```python
from build123d import *

# Parameters (mm, degrees)
SKETCH009_W     = 12.5
SKETCH009_H     = 5.72
PAD007_DEPTH    = 6.75
PAD008_DEPTH    = 0.5
POCKET002_DEPTH = 12


with BuildPart() as part:
    # Sketch009 → Pad007 (new body, symmetric)
    with BuildSketch(Plane.XZ):
        with Locations((0, 4.14)):
            Rectangle(SKETCH009_W, SKETCH009_H)
    extrude(amount=PAD007_DEPTH, both=True)

    # Sketch010 (on Face6 of Pad007) → Pad008 (join)
    with BuildSketch(Plane.XZ.offset(6.75)):
        with BuildLine():
            ThreePointArc((-6.75, 7.74), (-7.103553, 7.593553), (-7.25, 7.24))
            Line((-7.25, 1.04), (-7.25, 7.24))
            ThreePointArc((-7.25, 1.04), (-7.103553, 0.686447), (-6.75, 0.54))
            Line((6.75, 0.54), (-6.75, 0.54))
            ThreePointArc((6.75, 0.54), (7.103553, 0.686447), (7.25, 1.04))
            Line((7.25, 7.24), (7.25, 1.04))
            ThreePointArc((7.25, 7.24), (7.103553, 7.593553), (6.75, 7.74))
            Line((-6.75, 7.74), (6.75, 7.74))
        make_face()
    extrude(amount=PAD008_DEPTH)

    # Sketch011 (on Face5 of Pad008) → Pocket002 (cut)
    with BuildSketch(Plane.XZ.offset(7.25)):
        with BuildLine():
            ThreePointArc((-5.35, 6.29), (-5.703553, 6.143553), (-5.85, 5.79))
            Line((-5.85, 2.49), (-5.85, 5.79))
            ThreePointArc((-5.85, 2.49), (-5.703553, 2.136447), (-5.35, 1.99))
            Line((5.35, 1.99), (-5.35, 1.99))
            ThreePointArc((5.35, 1.99), (5.703553, 2.136447), (5.85, 2.49))
            Line((5.85, 5.79), (5.85, 2.49))
            ThreePointArc((5.85, 5.79), (5.703553, 6.143553), (5.35, 6.29))
            Line((-5.35, 6.29), (5.35, 6.29))
        make_face()
    extrude(amount=-POCKET002_DEPTH, mode=Mode.SUBTRACT)


with BuildPart() as part_1:
    # Body004 placement: moved
    add(part.part.moved(Location((-9.53, -23.5, 1.6))))


solid = part_1.part
```
Work out the finished part from the listing and answer in its coordinate system (mm). A direction names the side the tool comes from. Coordinates: 2 decimals unless noted, no trailing zeros. Write each loop counter-clockwise with the first axis right and the second up, starting at its lowest first coordinate (ties: lowest second). Pieces come first, ordered by that corner, then holes. Notation, with made-up numbers: (-38.75, 62.5) - (13.25, 62.5) arc R18 ccw to (13.25, 92.5) - close; hole circle Ø6 at (55, 38.25). An arc over 180 degrees is marked (long way). Answer as a JSON object with one key per item and string values.
Q1. Consider L1, parallel to Z at x = -14.25, y = -25.5; L2, parallel to X at y = -29.75, z = 5.5; L3, parallel to X at y = -26.25, z = 3.25. Determine where each line is inside the solid, lowest interval first. Write a range as from..to.
Results list:
{"L1": "z = 2.88..3.59, 7.89..8.6", "L2": "x = -15.78..-15.38, -3.68..-3.28", "L3": "x = -15.78..-3.28"}
Q2. Find section B-B (z = 4.5). Write down the section's boundary in (x, y), plus the area to 3 significant figures.
Results list:
{"outline": "(-16.78, -30.75) - (-15.38, -30.75) - (-15.38, -18.75) - (-3.68, -18.75) - (-3.68, -30.75) - (-2.28, -30.75) - (-2.28, -30.25) - (-3.28, -30.25) - (-3.28, -16.75) - (-15.78, -16.75) - (-15.78, -30.25) - (-16.78, -30.25) - close", "area": "35.6 mm^2"}
Q3. Find section D-D (y = -18). Write down the section's boundary in (x, z), plus the area to 3 significant figures.
Results list:
{"outline": "(-15.78, 2.88) - (-3.28, 2.88) - (-3.28, 8.6) - (-15.78, 8.6) - close", "area": "71.5 mm^2"}
Q4. Which of the six approach directions +Z, -Z, +X, -X, +Y, -Y give full straight-line access (tool end or side, diameter ignored) to faces 1 (the flat face through (-15.78, -24, 6)), 2 (the flat face through (-10, -25, 7.89)), 3 (the flat face through (-3.28, -24, 6)), 4 (the flat face through (-10, -24, 2.88))?
Results list:
{"face 1": "+Z, -Z, -X, +Y", "face 2": "-Y", "face 3": "+Z, -Z, +X, +Y", "face 4": "-Z, +X, -X, +Y"}
Q5. For a pull along Z with two mould halves and no side action, classify faces 5 (the flat face through (-10, -24, 8.6)), 6 (the flat face through (-10, -30.25, 9)), 7 (the flat face through (-15.38, -25, 6)) as pulls with the +Z half, pulls with the -Z half, needs draft (parallel to the pull), parting line crosses it, or undercut.
Results list:
{"face 5": "pulls with the +Z half", "face 6": "needs draft", "face 7": "undercut"}
Q6. Find section A-A (y = -23.5). Write down the section's boundary in (x, z).
Results list:
{"outline": "(-15.78, 2.88) - (-3.28, 2.88) - (-3.28, 8.6) - (-15.78, 8.6) - close; hole (-15.38, 4.09) arc R0.5 ccw to (-14.88, 3.59) - (-4.18, 3.59) arc R0.5 ccw to (-3.68, 4.09) - (-3.68, 7.39) arc R0.5 ccw to (-4.18, 7.89) - (-14.88, 7.89) arc R0.5 ccw to (-15.38, 7.39) - close"}
Q7. Given pin 1 Ø6 at (x, y) = (-6.5, -24) entering from -Z; pin 2 Ø6 at (x, y) = (-9, -26.5) entering from +Z; pin 3 Ø1.7 at (y, z) = (-20.5, 6) entering from +X, each flat-ended and moving along its own axis, determine where each tip first touches the part or whether it passes through.
Results list:
{"pin 1": "stops at z = 2.88", "pin 2": "stops at z = 8.6", "pin 3": "stops at x = -3.28"}
Q8. Find section C-C (x = -14.5). Write down the section's boundary in (y, z), plus the area to 3 significant figures.
Results list:
{"outline": "(-30.75, 2.14) - (-30.25, 2.14) - (-30.25, 2.88) - (-16.75, 2.88) - (-16.75, 8.6) - (-30.25, 8.6) - (-30.25, 9.34) - (-30.75, 9.34) - (-30.75, 7.89) - (-18.75, 7.89) - (-18.75, 3.59) - (-30.75, 3.59) - close", "area": "29.2 mm^2"}
